```python
from build123d import *

# Parameters (mm, degrees)
BASPROSKE_W             = 30
BASPROSKE_H             = 38.75
TOOTHCUT_DEPTH          = 63.474994998
TEETHCUTS_COUNT         = 29
TEETHCUTS_ANGLE         = 347.586206897
BORSKE_R                = 6
BORE_DEPTH              = 50.0000508
ESQUISSE1_R             = 4
BOSS_EXTRU_1_DEPTH      = 6
ESQUISSE2_R             = 11.5
ENL_V_MAT_EXTRU_1_DEPTH = 63.46458662
ESQUISSE3_R             = 23
ESQUISSE3_R_2           = 8
BOSS_EXTRU_2_DEPTH      = 5
ESQUISSE4_R             = 33
ESQUISSE4_R_2           = 8
BOSS_EXTRU_3_DEPTH      = 5


with BuildPart() as part:
    # BasProSke → Base-Revolve (revolve)
    with BuildSketch(Plane(origin=(0, 0, 0), x_dir=(1, 0, 0), z_dir=(0, 1, 0)), mode=Mode.PRIVATE) as base_revolve_sk:
        with Locations((15, 19.375)):
            Rectangle(BASPROSKE_W, BASPROSKE_H)
    revolve(base_revolve_sk.sketch.rotate(Axis((-10, 0, 0), (1, 0, 0)), 180), axis=Axis((-10, 0, 0), (1, 0, 0)))

    # TooCutSke → ToothCut (cut, through all)
    with BuildSketch(Plane(origin=(0, 0, 0), x_dir=(0, 0, -1), z_dir=(1, 0, 0))):
        with BuildLine():
            ThreePointArc((1.38827379, 33.094894952), (0, 33.124), (-1.38827379, 33.094894952))
            ThreePointArc((-1.38827379, 33.094894952), (-2.036611336, 35.961759797), (-3.249771531, 38.63897812))
            ThreePointArc((-3.249771531, 38.63897812), (0, 38.7754), (3.249771531, 38.63897812))
            ThreePointArc((3.249771531, 38.63897812), (2.036611336, 35.961759797), (1.38827379, 33.094894952))
        make_face()
    toothcut = extrude(amount=TOOTHCUT_DEPTH, mode=Mode.SUBTRACT)

    # TeethCuts: ToothCut ×29 about axis
    teethcuts_axis = Axis((-10, 0, 0), (1, 0, 0))
    for i in range(1, TEETHCUTS_COUNT):
        add(toothcut.rotate(teethcuts_axis, i * TEETHCUTS_ANGLE / (TEETHCUTS_COUNT - 1)), mode=Mode.SUBTRACT)

    # BorSke → Bore (cut, symmetric)
    with BuildSketch(Plane(origin=(0, 0, 0), x_dir=(0, 0, -1), z_dir=(1, 0, 0))):
        with Locations(Location((0, 0, 0), (0, 0, 180))):
            Circle(BORSKE_R)
    extrude(amount=BORE_DEPTH, both=True, mode=Mode.SUBTRACT)

    # Esquisse1 → Boss.-Extru.1 (add)
    with BuildSketch(Plane(origin=(30, 0, 0), x_dir=(0, 0, -1), z_dir=(1, 0, 0))):
        with Locations(Location((0, 25, 0), (0, 0, 180))):
            Circle(ESQUISSE1_R)
        with Locations(Location((-25, 0, 0), (0, 0, 180))):
            Circle(ESQUISSE1_R)
        with Locations(Location((25, 0, 0), (0, 0, 180))):
            Circle(ESQUISSE1_R)
        with Locations(Location((0, -25, 0), (0, 0, 180))):
            Circle(ESQUISSE1_R)
    extrude(amount=BOSS_EXTRU_1_DEPTH)

    # Esquisse2 → Enlèv. mat.-Extru.1 (cut, through all)
    with BuildSketch(Plane(origin=(30, 0, 0), x_dir=(0, 0, -1), z_dir=(1, 0, 0))):
        Circle(ESQUISSE2_R)
    extrude(amount=-ENL_V_MAT_EXTRU_1_DEPTH, mode=Mode.SUBTRACT)

    # Esquisse3 → Boss.-Extru.2 (add)
    with BuildSketch(Plane.ZY):
        with Locations(Location((0, 0, 0), (0, 0, 180))):
            Circle(ESQUISSE3_R)
        Circle(ESQUISSE3_R_2, mode=Mode.SUBTRACT)
    extrude(amount=BOSS_EXTRU_2_DEPTH)

    # Esquisse4 → Boss.-Extru.3 (add)
    with BuildSketch(Plane.ZY.offset(5)):
        Circle(ESQUISSE4_R)
        Circle(ESQUISSE4_R_2, mode=Mode.SUBTRACT)
    extrude(amount=BOSS_EXTRU_3_DEPTH)


solid = part.part
```
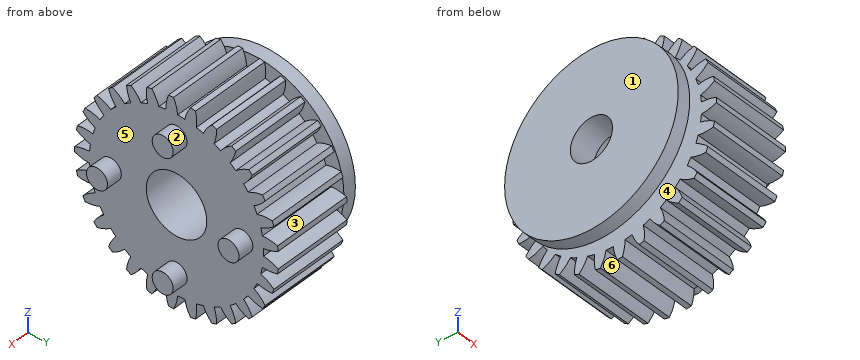
Verification items for the finished model (mm, model axes). Face numbers are marked on the shaded views. A direction names the side the tool comes from. Give positions to 0.01 mm unless a question says otherwise; leave off trailing zeros. Loops run counter-clockwise (first coordinate to the right, second up) from the corner with the lowest first, then second, coordinate; pieces in that order, holes last. Notation, with made-up numbers: M 66,13 L 83,13 A30 cw 83,36 Z; hole C 86.5,-33.75 d8. An arc over 180 degrees is marked long. Return JSON: item names as keys, results as strings.
1) Mould release check, pull along Y, two halves, no side actions. Record for the marked faces 1, 2 and 3: released by +Y, released by -Y, zero draft, split by the parting line, or undercut.
Findings:
{"face 1": "zero draft", "face 2": "split by the parting line", "face 3": "undercut"}
2) Material ranges on L1, parallel to X at y = 17, z = -20.5; L2, parallel to Z at x = 24.5, y = -17.5; L3, parallel to Z at x = 28, y = 12, recorded low to high. Write a range as [from, to].
Findings:
{"L1": "x = [-10, -5], [0, 30]", "L2": "z = [-34.57, -28.32], [-28.12, 28.12], [28.32, 34.57]", "L3": "z = [-34.69, 34.69]"}
3) Tool access check on the marked faces 4, 5 and 6. Record the directions out of +Z, -Z, +X, -X, +Y, -Y that give a thin tool (end or side, any length) a straight path to the whole face; none if there is none.
Findings:
{"face 4": "none", "face 5": "+X", "face 6": "-Z, +X, -X"}
4) Gauge pin test, flat ends, axial feed: P1, Ø10, axis at y = -22, z = -10, coming from the +X side; P2, Ø3, axis at x = 5, y = 28.5, coming from the +Z side; P3, Ø5, axis at y = 5, z = -4.5, coming from the +X side. Record the tip position at first contact, or that the pin passes through.
Findings:
{"P1": "stops at x = 30", "P2": "stops at z = 27.34", "P3": "stops at x = 0"}
5) Section check A-A, the plane z = 0. Enter the section's corners in (x, y), and give its area (3 significant figures).
Findings:
{"outline": "M -10,-33 L -5,-33 L -5,-23 L 0,-23 L 0,-38.75 L 30,-38.75 L 30,-29 L 36,-29 L 36,-21 L 30,-21 L 30,-11.5 L 0,-11.5 L 0,-8 L -10,-8 Z; M -10,8 L 0,8 L 0,11.5 L 30,11.5 L 30,21 L 36,21 L 36,29 L 30,29 L 30,33.12 L 0,33.12 L 0,23 L -5,23 L -5,33 L -10,33 Z", "area": "1,960 mm2"}
